CAD build for the part. Positions are in the model's coordinates, mm. A direction names the side the tool comes from. Give positions to 0.01 mm unless a question says otherwise; leave off trailing zeros. Loops run counter-clockwise (first coordinate to the right, second up) from the corner with the lowest first, then second, coordinate; pieces in that order, holes last.
```python
from build123d import *

# Parameters (mm, degrees)
BOSS_EXTRUDE1_DEPTH = 171.2
FILLET1_R           = 1
SKETCH2_R           = 1.8
CUT_EXTRUDE1_DEPTH  = 200
CUT_EXTRUDE2_DEPTH  = 2
LPATTERN1_COUNT     = 3
LPATTERN1_PITCH     = 116
CUT_EXTRUDE3_DEPTH  = 1
SKETCH5_W           = 10.598271306
SKETCH5_H           = 4.806690724
CUT_EXTRUDE4_DEPTH  = 16.6
SKETCH6_W           = 3
SKETCH6_H           = 2
CUT_EXTRUDE5_DEPTH  = 2
THICKEN1_T1         = 40


with BuildPart() as part:
    # Sketch1 → Boss-Extrude1 (new body)
    with BuildSketch(Plane.XY):
        Polygon((0, 0), (5.8, 0), (8.7, 3.9), (-2.9, 3.9), align=None)
    extrude(amount=BOSS_EXTRUDE1_DEPTH)

    # Fillet1
    fillet1_edges = [part.edges().sort_by_distance(p)[0] for p in [
        (-2.9, 3.9, 85.6),
        (8.7, 3.9, 85.6),
    ]]
    fillet(fillet1_edges, radius=FILLET1_R)

    # Sketch2 → Cut-Extrude1 (cut)
    with BuildSketch(Plane.XZ):
        with Locations(Location((2.9, 143.6, 0), (0, 0, 270))):
            Circle(SKETCH2_R)
    cut_extrude1 = extrude(amount=-CUT_EXTRUDE1_DEPTH, mode=Mode.SUBTRACT)

    # Sketch3 → Cut-Extrude2 (cut)
    with BuildSketch(Plane.XZ):
        Polygon((2.92874321, 146.948508199), (0.01447844, 145.29914645), (-0.014264771, 141.950638251), (2.87125679, 140.251491801), (5.78552156, 141.90085355), (5.814264771, 145.249361749), align=None)
    cut_extrude2 = extrude(amount=-CUT_EXTRUDE2_DEPTH, mode=Mode.SUBTRACT)

    # LPattern1: Cut-Extrude1, Cut-Extrude2 ×3
    with Locations(*[(0, 0, -i * LPATTERN1_PITCH) for i in range(1, LPATTERN1_COUNT)]):
        add(cut_extrude1, mode=Mode.SUBTRACT)
        add(cut_extrude2, mode=Mode.SUBTRACT)

    # Sketch4 → Cut-Extrude3 (cut)
    with BuildSketch(Plane(origin=(0, 3.9, 0), x_dir=(1, 0, 0), z_dir=(0, 1, 0))):
        with BuildLine():
            Line((0.677254142, -78.273076923), (-0.177553551, -78.273076923))
            add(Edge.make_bspline(
                [(-0.177553551, -78.273076923), (-0.154395416, -78.177194235), (-0.109123158, -77.989751421), (-0.01469619, -77.72194309), (0.088171783, -77.468514078), (0.211694989, -77.234209763), (0.346429527, -77.014321321), (0.500796362, -76.81383606), (0.667673607, -76.627655062), (0.852254362, -76.462428322), (1.045825934, -76.312810359), (1.251115864, -76.185243239), (1.463993881, -76.075503937), (1.685934908, -75.985097449), (1.917599703, -75.916992274), (2.156893893, -75.867579824), (2.404444561, -75.835491149), (2.572486218, -75.83235943), (2.657813036, -75.830769231)],
                knots=[0, 0, 0, 0, 1.162005537, 2.271625781, 3.343758855, 4.383309926, 5.390229558, 6.379919256, 7.361854164, 8.333198761, 9.295911338, 10.242430842, 11.177959212, 12.116337295, 13.062827104, 14.020064771, 14.994644689, 16, 16, 16, 16], degree=3))
            add(Edge.make_bspline(
                [(2.657813036, -75.830769231), (2.782135355, -75.834522707), (3.028068164, -75.841947786), (3.389373313, -75.909750646), (3.737789156, -76.017043327), (4.069502038, -76.165289685), (4.377617915, -76.348135158), (4.651764252, -76.565753478), (4.888225128, -76.813945863), (5.08660197, -77.088082341), (5.241927503, -77.381059121), (5.356462562, -77.682593834), (5.426190137, -77.991971199), (5.435226795, -78.200860651), (5.439754142, -78.305513822)],
                knots=[0, 0, 0, 0, 1.083050992, 2.142477498, 3.193116406, 4.255571735, 5.30263384, 6.308962982, 7.297363603, 8.282367274, 9.249857812, 10.179914175, 11.08814088, 12, 12, 12, 12], degree=3))
            add(Edge.make_bspline(
                [(5.439754142, -78.305513822), (5.436587512, -78.406225171), (5.430390908, -78.603301651), (5.37777561, -78.891015154), (5.289230494, -79.162182652), (5.166576355, -79.417945672), (5.007803993, -79.656682557), (4.815473296, -79.878930446), (4.588226767, -80.085675083), (4.416017657, -80.20411022), (4.32735931, -80.265084135)],
                knots=[0, 0, 0, 0, 1.024540389, 2.004866551, 2.965041327, 3.920577974, 4.882998113, 5.874504559, 6.905732034, 8, 8, 8, 8], degree=3))
            add(Edge.make_bspline(
                [(4.32735931, -80.265084135), (4.42868287, -80.314010444), (4.62943415, -80.410947615), (4.903075234, -80.601055069), (5.151481452, -80.820555557), (5.290012287, -80.991849491), (5.35961592, -81.077914663)],
                knots=[0, 0, 0, 0, 1.015518401, 2.012035669, 3.001164323, 4, 4, 4, 4], degree=3))
            add(Edge.make_bspline(
                [(5.35961592, -81.077914663), (5.405448431, -81.140664687), (5.496362912, -81.26513716), (5.608582472, -81.465261291), (5.710388704, -81.667603558), (5.789718944, -81.87758737), (5.85115211, -82.092778929), (5.895065169, -82.313547735), (5.922345153, -82.540074068), (5.926251905, -82.69332446), (5.92821568, -82.770357572)],
                knots=[0, 0, 0, 0, 1.025084078, 2.033381695, 3.024893161, 4.013698104, 4.991890475, 5.976764909, 6.982997093, 8, 8, 8, 8], degree=3))
            add(Edge.make_bspline(
                [(5.92821568, -82.770357572), (5.92333204, -82.903734028), (5.913587741, -83.169859267), (5.826490939, -83.563036902), (5.691472048, -83.947372019), (5.49972853, -84.314968546), (5.266046238, -84.658903726), (4.988032377, -84.966632824), (4.668845794, -85.231151883), (4.312867564, -85.452159718), (3.927194522, -85.628829206), (3.514692375, -85.751449818), (3.081304728, -85.83131286), (2.784104868, -85.839876839), (2.633008348, -85.844230769)],
                knots=[0, 0, 0, 0, 0.955779014, 1.907060117, 2.875433937, 3.871313158, 4.872415639, 5.851225146, 6.836215519, 7.83643374, 8.849228613, 9.86973379, 10.916971861, 12, 12, 12, 12], degree=3))
            add(Edge.make_bspline(
                [(2.633008348, -85.844230769), (2.531174395, -85.841867989), (2.330799134, -85.837218825), (2.036222185, -85.805436346), (1.75503956, -85.74738826), (1.486871083, -85.669274265), (1.231478519, -85.570236738), (0.989641205, -85.446905139), (0.75987128, -85.301821694), (0.544336992, -85.133273858), (0.343064032, -84.944729641), (0.161401262, -84.732841907), (-0.003680032, -84.501527543), (-0.147759642, -84.248099797), (-0.277400206, -83.975833776), (-0.384028381, -83.68124322), (-0.477878392, -83.366961703), (-0.52151232, -83.147947281), (-0.543899705, -83.035576923)],
                knots=[0, 0, 0, 0, 1.048658725, 2.063410685, 3.046034179, 4.001477787, 4.936774919, 5.862367409, 6.792675028, 7.730719943, 8.675894397, 9.627829632, 10.600096036, 11.597688215, 12.626045268, 13.701542398, 14.82072376, 16, 16, 16, 16], degree=3))
            Line((-0.543899705, -83.035576923), (0.310907988, -83.035576923))
            add(Edge.make_bspline(
                [(0.310907988, -83.035576923), (0.333178231, -83.108916738), (0.376495788, -83.251569048), (0.450230985, -83.456874451), (0.534236783, -83.645083153), (0.624355689, -83.817575792), (0.719002745, -83.976051116), (0.824906934, -84.116318631), (0.934224394, -84.244539288), (1.016627491, -84.316778554), (1.056956666, -84.352133413)],
                knots=[0, 0, 0, 0, 1.198163088, 2.33053128, 3.407730985, 4.417276592, 5.372219308, 6.28897303, 7.162600585, 8, 8, 8, 8], degree=3))
            add(Edge.make_bspline(
                [(1.056956666, -84.352133413), (1.110287349, -84.393249665), (1.216784096, -84.475355251), (1.390324782, -84.580134683), (1.572837079, -84.670924331), (1.768275585, -84.740276389), (1.972422925, -84.798998451), (2.188578826, -84.837426435), (2.414836267, -84.863792102), (2.56932568, -84.866118737), (2.648272771, -84.867307692)],
                knots=[0, 0, 0, 0, 0.946170439, 1.889420265, 2.845303464, 3.807233317, 4.801018734, 5.828864929, 6.890507805, 8, 8, 8, 8], degree=3))
            add(Edge.make_bspline(
                [(2.648272771, -84.867307692), (2.737409089, -84.86563155), (2.911707464, -84.862353999), (3.166038188, -84.832212254), (3.407993456, -84.788314486), (3.634886919, -84.720515583), (3.849690657, -84.636747694), (4.049393574, -84.531568819), (4.236617263, -84.408166398), (4.408963717, -84.267906259), (4.563936848, -84.114359191), (4.700387952, -83.953759333), (4.816387923, -83.786783825), (4.909960376, -83.612508653), (4.983848659, -83.431655495), (5.034149369, -83.243716823), (5.069123849, -83.050230692), (5.07197213, -82.918706855), (5.073407988, -82.852403846)],
                knots=[0, 0, 0, 0, 1.217147791, 2.380027433, 3.494444702, 4.572153297, 5.609568379, 6.639424714, 7.649109417, 8.668170816, 9.669597737, 10.625200337, 11.543417969, 12.441394052, 13.322311151, 14.205496177, 15.095365482, 16, 16, 16, 16], degree=3))
            add(Edge.make_bspline(
                [(5.073407988, -82.852403846), (5.069243381, -82.763654417), (5.060934891, -82.586597163), (4.997502257, -82.326108621), (4.893165777, -82.075129192), (4.747099871, -81.837940935), (4.569293352, -81.618115088), (4.361471713, -81.421977697), (4.121909177, -81.260134092), (3.901419391, -81.148314248), (3.706115643, -81.072013351), (3.538978061, -81.021190769), (3.351861877, -80.978155035), (3.147029884, -80.938116639), (2.922938702, -80.904040684), (2.679832296, -80.875624028), (2.417661402, -80.852886381), (2.236166158, -80.842732472), (2.142638757, -80.8375)],
                knots=[0, 0, 0, 0, 1.07054697, 2.135767047, 3.216561865, 4.33974944, 5.486079747, 6.621378074, 7.775625952, 8.963672916, 9.598146892, 10.304877434, 11.070270905, 11.915000392, 12.823868403, 13.805723172, 14.86925407, 16, 16, 16, 16], degree=3))
            Line((2.142638757, -80.8375), (2.142638757, -79.860576923))
            add(Edge.make_bspline(
                [(2.142638757, -79.860576923), (2.260479787, -79.858577207), (2.491301415, -79.854660255), (2.828470916, -79.807285598), (3.150887573, -79.741751889), (3.451406063, -79.641371473), (3.725314348, -79.524784665), (3.962948408, -79.389115438), (4.160979001, -79.238308156), (4.318443774, -79.070035126), (4.436905461, -78.889563461), (4.523519817, -78.701467414), (4.574683562, -78.504098363), (4.581513441, -78.369402159), (4.584946449, -78.301697716)],
                knots=[0, 0, 0, 0, 1.321986639, 2.589447074, 3.816329219, 5.01088745, 6.139805852, 7.153945165, 8.075214402, 8.924034688, 9.728124013, 10.488707548, 11.240355623, 12, 12, 12, 12], degree=3))
            add(Edge.make_bspline(
                [(4.584946449, -78.301697716), (4.583818659, -78.251956138), (4.581574975, -78.152997628), (4.553279526, -78.008421549), (4.510759815, -77.868265403), (4.452304266, -77.733125219), (4.374062653, -77.60393826), (4.280429219, -77.479603131), (4.16893746, -77.360829704), (4.041178779, -77.25012112), (3.903986653, -77.14461341), (3.753628337, -77.055041298), (3.594637377, -76.978446522), (3.426837753, -76.91528352), (3.249684916, -76.867769314), (3.064011213, -76.833653917), (2.869462589, -76.812324299), (2.736733804, -76.809253396), (2.669261353, -76.807692308)],
                knots=[0, 0, 0, 0, 0.884392785, 1.759457502, 2.611959086, 3.489218968, 4.37281399, 5.2945488, 6.255912374, 7.266815255, 8.301784654, 9.332968512, 10.37626691, 11.440494194, 12.520033166, 13.637162961, 14.798855837, 16, 16, 16, 16], degree=3))
            add(Edge.make_bspline(
                [(2.669261353, -76.807692308), (2.560807885, -76.8114788), (2.348973038, -76.8188747), (2.043588157, -76.883652901), (1.759690541, -76.987007543), (1.542687455, -77.110378117), (1.382442736, -77.232163226), (1.267933354, -77.338523149), (1.155482536, -77.456722476), (1.05248823, -77.59404134), (0.948328336, -77.741180248), (0.853501351, -77.905618981), (0.761354617, -78.083068083), (0.705830536, -78.20851406), (0.677254142, -78.273076923)],
                knots=[0, 0, 0, 0, 1.472543308, 2.876219568, 4.221790263, 5.565193594, 6.249813518, 6.953379497, 7.687249741, 8.463570142, 9.283606569, 10.136032583, 11.040678096, 12, 12, 12, 12], degree=3))
        make_face()
    extrude(amount=-CUT_EXTRUDE3_DEPTH, mode=Mode.SUBTRACT)

    # Sketch5 → Cut-Extrude4 (cut)
    with BuildSketch(Plane.XY.offset(171.2)):
        with Locations((3.01775857, 2.046347921)):
            Rectangle(SKETCH5_W, SKETCH5_H)
    extrude(amount=-CUT_EXTRUDE4_DEPTH, mode=Mode.SUBTRACT)

    # Sketch6 → Cut-Extrude5 (cut)
    with BuildSketch(Plane(origin=(0, 3.9, 0), x_dir=(1, 0, 0), z_dir=(0, 1, 0))):
        with Locations((2.9, -154.6)):
            Rectangle(SKETCH6_W, SKETCH6_H)
    extrude(amount=-CUT_EXTRUDE5_DEPTH, mode=Mode.SUBTRACT)

    # Surface-Offset1: a surface, a copy of 1 face of the part
    surface_offset1_1 = part.part.faces().sort_by_distance((2.9, 2.093393293, 0))[0]
    add(Solid.thicken(surface_offset1_1, THICKEN1_T1))


solid = part.part
```
1. Tool access for faces 1 (the face through (4, 2.9, 81)), 2 (the face through (3, 3.9, 59)), 3 (the face through (1.56, 2, 26.16)): list every direction of +Z, -Z, +X, -X, +Y, -Y with a clear straight run to the whole face (end or side of a thin tool).
Responses:
face 1: +Y
face 2: +Z, -Z, +X, -X, +Y
face 3: -Y
2. Saw through at A-A, the plane z = -7. List the corners of the cut face in (x, y), and give its area (3 significant figures).
Responses:
outline: (-1.71, 2.3) - (0, 0) - (5.8, 0) - (7.51, 2.3) arc R1 ccw to (6.71, 3.9) - (-0.91, 3.9) arc R1 ccw to start
area: 32.2 mm2
3. Probe line 1 along Z through (x, y) = (3, 2.8); line 2 along Z through (x, y) = (3.25, 1.6); line 3 along X through (y, z) = (2.95, 143.6). List the from-to ranges inside material, lowest first.
Responses:
line 1: z = -40 to 25.8, 29.4 to 141.8, 145.4 to 153.6
line 2: z = -40 to 24.47, 30.76 to 140.47, 146.76 to 154.6
line 3: x = -1.91 to 1.1, 4.7 to 7.71
4. Drop flat-ended pins along their axis: pin 1 (0.5 mm diameter, centred on x = 3, z = 154, fed in from +Y); pin 2 (0.8 mm diameter, centred on y = 3.5, z = 80, fed in from +X); pin 3 (4.5 mm diameter, centred on x = 3.5, z = 27.5, fed in from -Y). Give the stop position or say it passes through.
Responses:
pin 1: stops at y = 1.9
pin 2: stops at x = 7.69
pin 3: stops at y = 2
5. Pull direction X, two halves, no side cores. Call faces 4 (the face through (1.56, 2, 142.16)), 5 (the face through (3, 0, -7)): released by +X, released by -X, zero draft, split by the parting line, or undercut.
Responses:
face 4: undercut
face 5: zero draft
